Check sheet for the modelled part. Datum: model origin and axes. Units: mm. A direction names the side the tool comes from. Coordinates: 2 decimals unless noted, no trailing zeros. Loops run counter-clockwise (first coordinate to the right, second up) from the corner with the lowest first, then second, coordinate; pieces in that order, holes last.
```python
from build123d import *

# Parameters (mm, degrees)
SKETCH1_R               = 1.25
BOSS_EXTRUDE1_DEPTH     = 2
BOSS_EXTRUDE2_DEPTH     = 7.5
SKETCH3_R               = 1.25
CUT_EXTRUDE1_DEPTH      = 2
CUT_EXTRUDE1_DEPTH_BACK = 4
SKETCH4_W               = 5
SKETCH4_H               = 2
SKETCH4_W_2             = 4.4
SKETCH4_H_2             = 1.4
CUT_EXTRUDE2_DEPTH      = 4


with BuildPart() as part:
    # Sketch1 → Boss-Extrude1 (new body)
    with BuildSketch(Plane.XY):
        Polygon((1952.176808721, 1466.884115951), (1957.176808721, 1466.884115951), (1957.176808721, 1462.884115951), (1958.426808721, 1462.884115951), (1958.426808721, 1458.884115951), (1957.176808721, 1458.884115951), (1957.176808721, 1454.884115951), (1952.176808721, 1454.884115951), (1952.176808721, 1458.884115951), (1950.926808721, 1458.884115951), (1950.926808721, 1462.884115951), (1952.176808721, 1462.884115951), align=None)
        with Locations((1954.676808721, 1460.884115951)):
            Circle(SKETCH1_R, mode=Mode.SUBTRACT)
    extrude(amount=BOSS_EXTRUDE1_DEPTH)

    # Sketch2 → Boss-Extrude2 (add)
    with BuildSketch(Plane.ZY.offset(-1950.926808721)):
        with BuildLine():
            Line((2, 1458.884115951), (2, 1459.884115951))
            ThreePointArc((2, 1459.884115951), (2.292893219, 1459.17700917), (3, 1458.884115951))
            Line((3, 1458.884115951), (2, 1458.884115951))
        make_face()
        with BuildLine():
            Line((0, 1458.884115951), (-1, 1458.884115951))
            ThreePointArc((-1, 1458.884115951), (-0.292893219, 1459.17700917), (0, 1459.884115951))
            Line((0, 1459.884115951), (0, 1458.884115951))
        make_face()
    extrude(amount=-BOSS_EXTRUDE2_DEPTH)

    # Sketch3 → Cut-Extrude1 (cut, two sides)
    with BuildSketch(Plane.XY.offset(2)) as cut_extrude1_sk:
        with Locations((1954.676808721, 1460.884115951)):
            Circle(SKETCH3_R)
    extrude(amount=CUT_EXTRUDE1_DEPTH, mode=Mode.SUBTRACT)
    extrude(cut_extrude1_sk.sketch, amount=-CUT_EXTRUDE1_DEPTH_BACK, mode=Mode.SUBTRACT)

    # Sketch4 → Cut-Extrude2 (cut)
    with BuildSketch(Plane(origin=(0, 1466.884115951, 0), x_dir=(1, 0, 0), z_dir=(0, 1, 0))):
        with Locations((1954.676808721, -1)):
            Rectangle(SKETCH4_W, SKETCH4_H)
        with Locations((1954.676808721, -1)):
            Rectangle(SKETCH4_W_2, SKETCH4_H_2, mode=Mode.SUBTRACT)
    extrude(amount=-CUT_EXTRUDE2_DEPTH, mode=Mode.SUBTRACT)


solid = part.part
```
1) Mould release check, pull along X, two halves, no side actions. Record for faces 5 (the cylindrical face through (1953.685, 1460.124, 0.986)), 6 (the flat face through (1952.477, 1465, 1)), 7 (the flat face through (1955, 1457, 2)): +X half, -X half, draft (parallel to the pull), parting line (faces both ways), or undercut.
Answer sheet:
face 5: undercut
face 6: -X half
face 7: draft
2) Section check A-A on x = 1955. Enter the section's corners in (y, z).
Answer sheet:
outline: (1454.88, 0) - (1458.88, 0) - (1458.88, -1) arc R1 cw to (1459.68, -0.02) - (1459.68, 2.02) arc R1 cw to (1458.88, 3) - (1458.88, 2) - (1454.88, 2) - close; (1462.09, 0) - (1462.88, 0) - (1462.88, 0.3) - (1466.88, 0.3) - (1466.88, 1.7) - (1462.88, 1.7) - (1462.88, 2) - (1462.09, 2) - close
3) Depth check by flat-ended pin: pin 1 (3 mm diameter, centred on x = 1956.5, y = 1463.5, fed in from -Z); pin 2 (1.2 mm diameter, centred on x = 1955.5, y = 1465.5, fed in from -Z); pin 3 (1.1 mm diameter, centred on y = 1464.5, z = 1.5, fed in from +X). Enter the tip coordinate at first touch or a pass-through.
Answer sheet:
pin 1: stops at z = 0
pin 2: stops at z = 0.3
pin 3: stops at x = 1956.88
4) Section check D-D on y = 1462.75. Enter the section's corners in (x, z).
Answer sheet:
outline: (1950.93, 0) - (1958.43, 0) - (1958.43, 2) - (1950.93, 2) - close
5) Section check C-C on x = 1952.75. Enter the section's corners in (y, z).
Answer sheet:
outline: (1454.88, 0) - (1458.88, 0) - (1458.88, -1) arc R1 cw to (1459.88, 0) - (1462.88, 0) - (1462.88, 0.3) - (1466.88, 0.3) - (1466.88, 1.7) - (1462.88, 1.7) - (1462.88, 2) - (1459.88, 2) arc R1 cw to (1458.88, 3) - (1458.88, 2) - (1454.88, 2) - close
6) Scan lines: line 1 (X direction, y = 1457, z = 0.7); line 2 (Y direction, x = 1953, z = 0.05); line 3 (Z direction, x = 1956.5, y = 1462.5). Record each from-to range of solid material in increasing order.
Answer sheet:
line 1: x = 1952.18 to 1957.18
line 2: y = 1454.88 to 1462.88
line 3: z = 0 to 2
7) Section check B-B on z = 1.85. Enter the section's corners in (x, y), plus the area to 3 significant figures.
Answer sheet:
outline: (1950.93, 1458.88) - (1952.18, 1458.88) - (1952.18, 1454.88) - (1957.18, 1454.88) - (1957.18, 1458.88) - (1958.43, 1458.88) - (1958.43, 1462.88) - (1950.93, 1462.88) - close; hole circle Ø2.5 at (1954.68, 1460.88)
area: 45.1 mm2
8) Set-up check for faces 1 (the flat face through (1952.177, 1457, 1)), 2 (the flat face through (1956.877, 1465, 1)), 3 (the flat face through (1955, 1465, 0.3)), 4 (the flat face through (1955, 1457, 0)): record each of +Z, -Z, +X, -X, +Y, -Y from which the full face is reachable in a straight line by a thin tool's end or side.
Answer sheet:
face 1: +Z, -Z, -X, -Y
face 2: +Z, -Z, +X, +Y
face 3: -Z, +X, -X, +Y
face 4: -Z, +X, -X, -Y
